Autodesk Inventor part; units mm, degrees
ref_plane "YZ Plane" through (0, 0, 0) normal (1, 0, 0) x (0, 1, 0)
ref_plane "XZ Plane" through (0, 0, 0) normal (0, 1, 0) x (-1, 0, 0)
ref_plane "XY Plane" through (0, 0, 0) normal (0, 0, 1) x (1, 0, 0)
sketch "草图1" plane through (0, 0, 0) normal (0, 1, 0) x (-1, 0, 0)
  line L0 (-150, -50) -> (150, -50)
  line L1 (150, -50) -> (150, 50)
  line L2 (150, 50) -> (-150, 50)
  line L3 (-150, 50) -> (-150, -50)
  line L4 (-150, -50) -> (150, 50) construction
  line L5 (150, -50) -> (-150, 50) construction
  point P0 (0, 0)
  dimension "d0" = 300
  dimension "d1" = 100
extrude "拉伸1" add sketch "草图1" along normal mid plane 10
sketch "草图2" plane through (0, 5, 0) normal (0, 1, 0) x (1, 0, 0)
  line L0 (-150, 50) -> (-150, -50)
  line L1 (150, -2.5) -> (-150, -2.5)
  line L2 (-150, -2.5) -> (-150, 2.5)
  line L3 (-150, 2.5) -> (150, 2.5)
  line L4 (150, 2.5) -> (150, -2.5)
  line L5 (150, -2.5) -> (-150, 2.5) construction
  line L6 (-150, -2.5) -> (150, 2.5) construction
  point P0 (0, 0)
  dimension "d4" = 5
extrude "拉伸2" cut sketch "草图2" against normal blind 5
sketch "草图3" plane through (0, -5, 0) normal (0, -1, 0) x (1, 0, 0)
  line L0 (-150, 50) -> (150, 50)
  line L1 (150, -50) -> (-150, -50)
  line L2 (150, 50) -> (140, 50)
  line L3 (140, 50) -> (140, -50)
  line L4 (140, -50) -> (150, -50)
  line L5 (150, -50) -> (150, 50)
  point P0 (0, 0)
extrude "拉伸3" add sketch "草图3" along normal blind 100
sketch "草图4" plane through (140, -5, -50) normal (-1, 0, 0) x (0, 0, 1)
  line L0 (100, 10) -> (100, -100)
  line L1 (100, 0) -> (0, 0)
  line L2 (100, -100) -> (90, -100)
  line L3 (90, -100) -> (90, 0)
  line L4 (90, 0) -> (100, 0)
  line L5 (100, 0) -> (100, -100)
  line L6 (0, -100) -> (0, 10)
  line L7 (0, -100) -> (10, -100)
  line L8 (10, -100) -> (10, 0)
  line L9 (10, 0) -> (0, 0)
  line L10 (0, 0) -> (0, -100)
  point P0 (50, 5)
extrude "拉伸4" add sketch "草图4" along normal blind 290
fillet "圆角1" radius 5 7 edges at (-150, -55, 40) (-150, -50, 50) (-150, -55, -40) (-150, -50, -50) (-150, -5, 0) (-150, 5, -26.25) (-150, 5, 26.25)
properties part number "滑盖上"
Model file for the job. Use its own axes, mm. A direction names the side the tool comes from. Give positions to 0.01 mm unless a question says otherwise; leave off trailing zeros. Loops run counter-clockwise (first coordinate to the right, second up) from the corner with the lowest first, then second, coordinate; pieces in that order, holes last. Notation, with made-up numbers: (9.5, 66.5) -> (22.5, 66.5) arc R14 cw to (22.5, 72.5) -> close; hole circle Ø8 at (89, 36). An arc over 180 degrees is marked (long way). Use a Markdown table: item, result. Add a question column.
(1) Drop flat-ended pins along their axis: pin 1 Ø1.5 at (y, z) = (-22, -1) entering from -X; pin 2 Ø10 at (x, z) = (50, -34.5) entering from -Y. Give the stop position or say it passes through.
(2) Slice it at A-A on x = -23.5. List the corners of the cut face in (y, z).
(3) Tool access for faces 4 (the flat face through (5, 5, -26)), 5 (the flat face through (-1, -56, 40)): list every direction of +Z, -Z, +X, -X, +Y, -Y with a clear straight run to the whole face (end or side of a thin tool).
(4) Wall check: line 1 along Z through (x, y) = (-91.5, -45); line 2 along X through (y, z) = (-36, 24.5); line 3 along Y through (x, z) = (-136.5, -38.5). Give the ranges that are in metal, low to high.
(5) Mould opens along Z. For faces 1 (the flat face through (-1, -56, -40)), 2 (the flat face through (5, -49, -50)), 3 (the flat face through (150, -49, -1)) say: +Z half, -Z half, draft (parallel to the pull), parting line (faces both ways), or undercut.
Filled sheet:
| question | item | result |
|---|---|---|
| 1 | pin 1 | x = 140 |
| 1 | pin 2 | y = -5 |
| 2 | outline | (-105, -50) -> (5, -50) -> (5, -2.5) -> (0, -2.5) -> (0, 2.5) -> (5, 2.5) -> (5, 50) -> (-105, 50) -> (-105, 40) -> (-5, 40) -> (-5, -40) -> (-105, -40) -> close |
| 3 | face 4 | +Z, -Z, +X, -X, +Y |
| 3 | face 5 | -X, -Y |
| 4 | line 1 | -50 to -40, 40 to 50 |
| 4 | line 2 | 140 to 150 |
| 4 | line 3 | -5 to 5 |
| 5 | face 1 | undercut |
| 5 | face 2 | -Z half |
| 5 | face 3 | draft |
